from build123d import *

# Parameters (mm, degrees)
F0_R     = 6
F1_DEPTH = 10
F2_R     = 5
F4_D     = 6
F5_D     = 6


with BuildPart() as f1:
    # F0 (on Right) → F1 (new body)
    with BuildSketch(Plane.YZ):
        with BuildLine():
            Line((20, -30), (20, 30))
            Line((20, 30), (-20, 30))
            Line((-20, 30), (-20, 10))
            Line((-20, 10), (-30, 10))
            ThreePointArc((-30, 10), (-40, 0), (-30, -10))
            Line((-30, -10), (-20, -10))
            Line((-20, -10), (-20, -30))
            Line((-20, -30), (20, -30))
        make_face()
        with Locations((-30, 0)):
            Circle(F0_R, mode=Mode.SUBTRACT)
    extrude(amount=F1_DEPTH)

    # F2
    f2_edges = [f1.edges().sort_by_distance(p)[0] for p in [
        (5, 20, 30),
        (5, 20, -30),
        (5, -20, 30),
        (5, -20, -30),
        (5, -20, -10),
        (5, -20, 10),
    ]]
    fillet(f2_edges, radius=F2_R)

    # F4 (through all)
    with Locations(Plane(origin=(0, 0, 0), x_dir=(0, -1, 0), z_dir=(-1, 0, 0))):
        with Locations((-10, -20), (10, -20)):
            Hole(F4_D / 2)

    # F5 (through all)
    with Locations(Plane(origin=(0, 0, 0), x_dir=(0, -1, 0), z_dir=(-1, 0, 0))):
        with Locations((10, 20), (-10, 20)):
            Hole(F5_D / 2)


solid = f1.part
Source: CAD feature listing. Evaluate the final solid. Frame: model axes, mm. A direction names the side the tool comes from. Give positions to 0.01 mm unless a question says otherwise; leave off trailing zeros. Write each loop counter-clockwise with the first axis right and the second up, starting at its lowest first coordinate (ties: lowest second). Pieces come first, ordered by that corner, then holes. Notation, with made-up numbers: (11.5, 23) - (55.5, 23) arc R18 ccw to (55.5, 54) - close; hole circle Ø2 at (-24.5, 37). An arc over 180 degrees is marked (long way). Write item = value, one per line. Start each with the question number.
Q1. Material intervals for probe 1 along Z at (x, y) = (4, -10); probe 2 along Y at (x, z) = (9.5, 19.5); probe 3 along Z at (x, y) = (9, -30), sorted ascending.
Q2. Draft query along Y for faces 4 (the flat face through (5, 20, 0)), 5 (the cylindrical face through (5.1, -12.4, 18.2)), 6 (the flat face through (5, -20, 20)), 7 (the flat face through (5, 0, 30)). Return one class per face: +Y half, -Y half, draft (parallel to the pull), parting line (faces both ways), or undercut.
Q3. Cut plane D-D, the plane z = 20. Return loops of the section in (x, y), then the cut area to 3 significant figures.
Q4. Cut plane B-B, the plane z = 0. Return loops of the section in (x, y).
Q5. Reachability of faces 1 (the flat face through (5, -27, 10)), 2 (the flat face through (5, -28, -10)), 3 (the cylindrical face through (5, 19, 28)) from +Z, -Z, +X, -X, +Y, -Y: full face, straight path, thin tool, end or side. Return the list, or none.
Q6. Pin query (flat end, axial travel): pin 1 Ø2 at (y, z) = (9, 19.5) entering from -X; pin 2 Ø4 at (x, y) = (5, -28) entering from +Z; pin 3 Ø5 at (x, z) = (9, -22) entering from -Y; pin 4 Ø7 at (y, z) = (10, 20) entering from -X. Return the tip coordinate at first contact, or that it passes through.
Q7. Cut plane C-C, the plane x = 6.75. Return loops of the section in (y, z).
Q8. Cut plane A-A, the plane y = -10. Return loops of the section in (x, z), then the cut area to 3 significant figures.
Computed values:
q1.probe_1 = -30 to -23, -17 to 17, 23 to 30
q1.probe_2 = -20 to -12.96, -7.04 to 7.04, 12.96 to 20
q1.probe_3 = -10 to -6, 6 to 10
q2.face_4 = +Y half
q2.face_5 = undercut
q2.face_6 = -Y half
q2.face_7 = draft
q3.outline = (0, -20) - (10, -20) - (10, -13) - (0, -13) - close; (0, -7) - (10, -7) - (10, 7) - (0, 7) - close; (0, 13) - (10, 13) - (10, 20) - (0, 20) - close
q3.area = 280 mm²
q4.outline = (0, -40) - (10, -40) - (10, -36) - (0, -36) - close; (0, -24) - (10, -24) - (10, 20) - (0, 20) - close
q5.face_1 = +Z, +X, -X, -Y
q5.face_2 = -Z, +X, -X, -Y
q5.face_3 = +Z, +X, -X, +Y
q6.pin_1 = through
q6.pin_2 = 10
q6.pin_3 = -20
q6.pin_4 = 0
q7.outline = (-30, -10) - (-25, -10) arc R5 cw to (-20, -15) - (-20, -25) arc R5 ccw to (-15, -30) - (15, -30) arc R5 ccw to (20, -25) - (20, 25) arc R5 ccw to (15, 30) - (-15, 30) arc R5 ccw to (-20, 25) - (-20, 15) arc R5 cw to (-25, 10) - (-30, 10) arc R10 ccw to start; hole circle Ø12 at (-30, 0); hole circle Ø6 at (-10, -20); hole circle Ø6 at (-10, 20); hole circle Ø6 at (10, -20); hole circle Ø6 at (10, 20)
q8.outline = (0, -30) - (10, -30) - (10, -23) - (0, -23) - close; (0, -17) - (10, -17) - (10, 17) - (0, 17) - close; (0, 23) - (10, 23) - (10, 30) - (0, 30) - close
q8.area = 480 mm²
